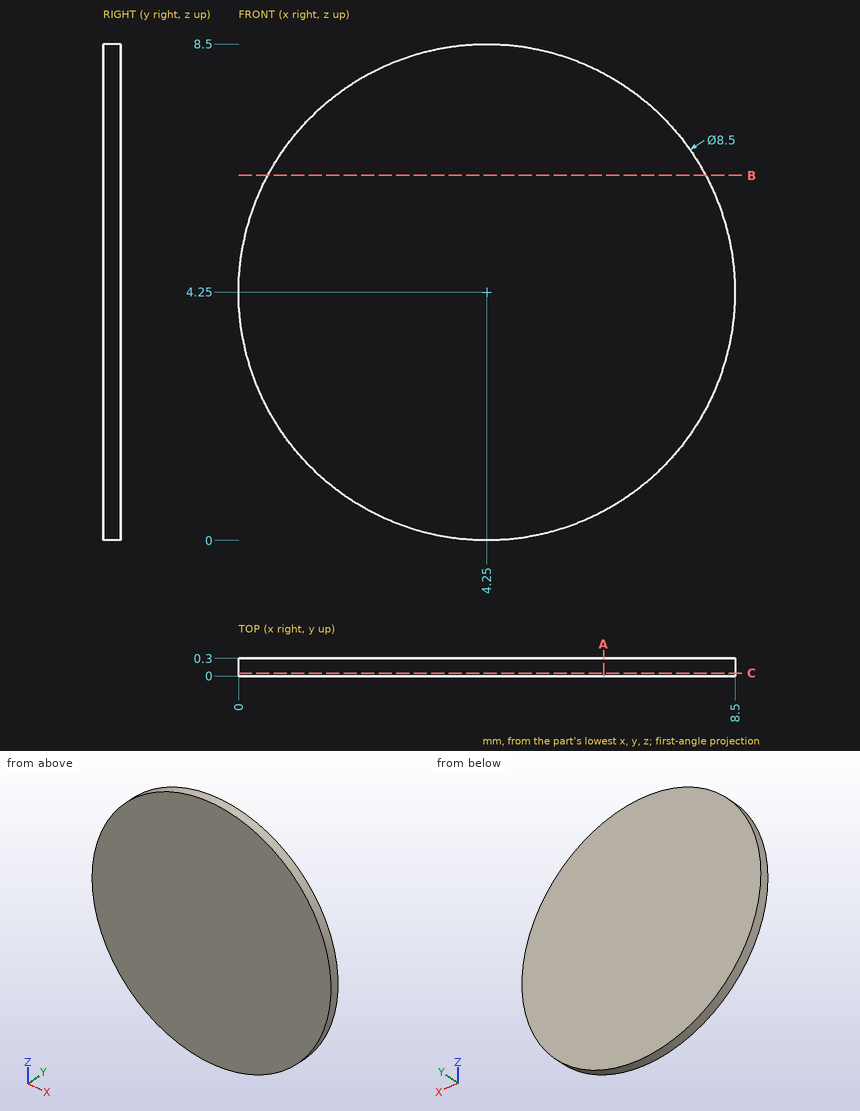
Verification items for this drawing (mm, ordinates from the low corner). Coordinates: 2 decimals unless noted, no trailing zeros. Loops run counter-clockwise (first coordinate to the right, second up) from the corner with the lowest first, then second, coordinate; pieces in that order, holes last. Notation, with made-up numbers: (-38, 5.25) - (8, 5.25) arc R22 ccw to (8, 20.25) - close; hole circle Ø11 at (-30, 19.5). An arc over 180 degrees is marked (long way). One line per item, written item: value. Start each with the question number.
(1) Cross-section at B-B on z = 6.25. Enter the section's corners in (x, y).
(2) Cross-section at A-A on x = 6.25. Enter the section's corners in (y, z).
(3) Depth check by flat-ended pin: P1, Ø2, axis at x = 1, z = 1.5, coming from the -Y side. Enter the tip coordinate at first touch or a pass-through.
(4) Material ranges on line 1 (X direction, y = 0.1, z = 6.75); line 2 (X direction, y = 0.15, z = 3.5); line 3 (Z direction, x = 2, y = 0.25), recorded low to high. Write a range as [from, to].
(5) Cross-section at C-C on y = 0.05. Enter the section's corners in (x, z).
Results below:
1. outline: (0.5, 0) - (8, 0) - (8, 0.3) - (0.5, 0.3) - close
2. outline: (0, 0.5) - (0.3, 0.5) - (0.3, 8) - (0, 8) - close
3. P1: stops at y = 0
4. line 1: x = [0.81, 7.69]
4. line 2: x = [0.07, 8.43]
4. line 3: z = [0.64, 7.86]
5. outline: circle Ø8.5 at (4.25, 4.25)
